Verification items for this drawing (mm, ordinates from the low corner). Give positions to 0.01 mm unless a question says otherwise; leave off trailing zeros. Loops run counter-clockwise (first coordinate to the right, second up) from the corner with the lowest first, then second, coordinate; pieces in that order, holes last. Notation, with made-up numbers: M -24,87.5 L -16,87.5 A17 cw -16,95.5 Z; hole C 89.5,17 d5. An arc over 180 degrees is marked long. Answer in a Markdown table with one row per item.
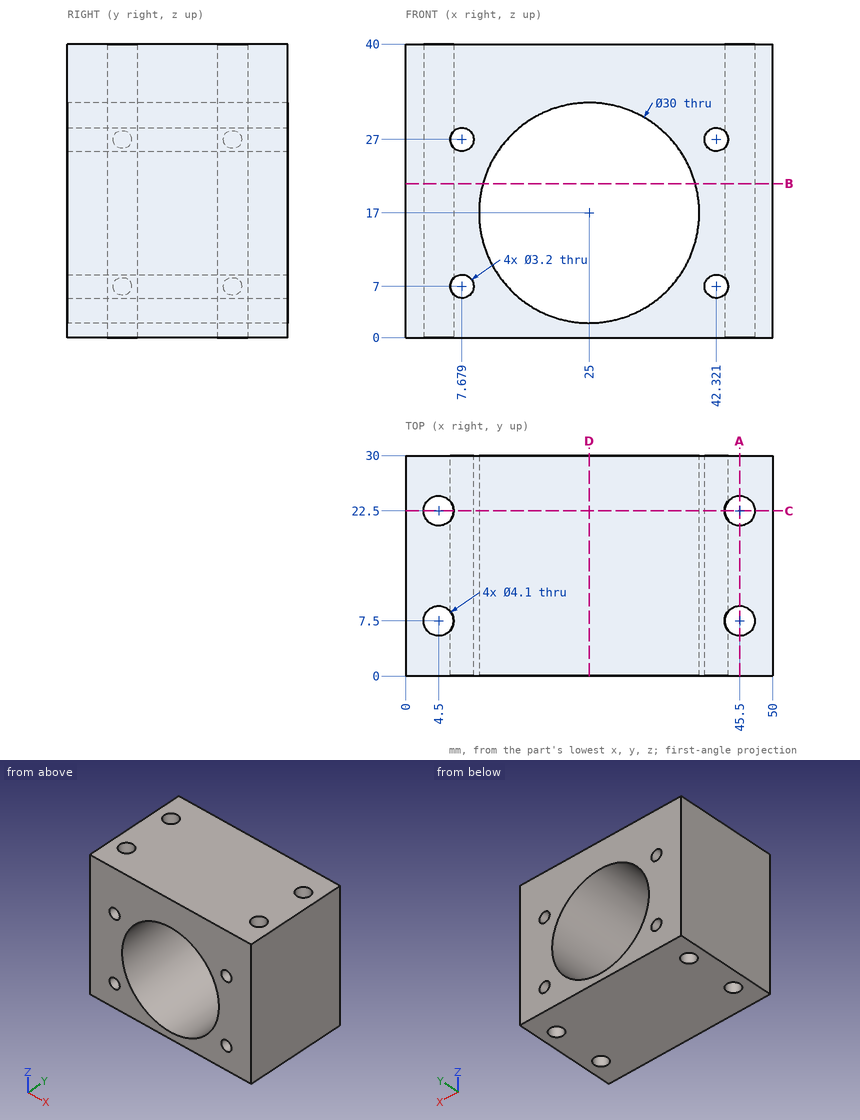
Item 1: Scan lines: L1, parallel to Z at x = 25, y = 4; L2, parallel to X at y = 23.5, z = 17.5; L3, parallel to Y at x = 45, z = 35. Record each from-to range of solid material in increasing order. Write a range as [from, to].
Reported:
| item | result |
|---|---|
| L1 | z = [0, 2], [32, 40] |
| L2 | x = [0, 2.71], [6.29, 10.01], [39.99, 43.71], [47.29, 50] |
| L3 | y = [0, 5.51], [9.49, 20.51], [24.49, 30] |
Item 2: Sectioned sample at A-A (x = 45.5). Record the cut outline in (y, z), and give its area (3 significant figures).
Reported:
| item | result |
|---|---|
| outline | M 0,0 L 5.45,0 L 5.45,40 L 0,40 Z; M 9.55,0 L 20.45,0 L 20.45,40 L 9.55,40 Z; M 24.55,0 L 30,0 L 30,40 L 24.55,40 Z |
| area | 872 mm^2 |
Item 3: Go/stop test with flat-tipped pins: pin 1 (3.5 mm diameter, centred on x = 42.32, z = 7, fed in from -Y); pin 2 (3 mm diameter, centred on x = 42.32, z = 27, fed in from +Y). Record where each tip stops, or that it passes through.
Reported:
| item | result |
|---|---|
| pin 1 | stops at y = 0 |
| pin 2 | passes through |
Item 4: Sectioned sample at C-C (y = 22.5). Record the cut outline in (x, z).
Reported:
| item | result |
|---|---|
| outline | M 0,0 L 2.45,0 L 2.45,40 L 0,40 Z; M 6.55,0 L 43.45,0 L 43.45,5.87 A1.6 cw long 43.45,8.13 L 43.45,25.87 A1.6 cw long 43.45,28.13 L 43.45,40 L 6.55,40 L 6.55,28.13 A1.6 cw long 6.55,25.87 L 6.55,8.13 A1.6 cw long 6.55,5.87 Z; M 47.55,0 L 50,0 L 50,40 L 47.55,40 Z; hole C 25,17 d30 |
Item 5: Sectioned sample at D-D (x = 25). Record the cut outline in (y, z), and give its area (3 significant figures).
Reported:
| item | result |
|---|---|
| outline | M 0,0 L 30,0 L 30,2 L 0,2 Z; M 0,32 L 30,32 L 30,40 L 0,40 Z |
| area | 300 mm^2 |
Item 6: Sectioned sample at B-B (z = 21). Record the cut outline in (x, y).
Reported:
| item | result |
|---|---|
| outline | M 0,0 L 10.54,0 L 10.54,30 L 0,30 Z; M 39.46,0 L 50,0 L 50,30 L 39.46,30 Z; hole C 4.5,7.5 d4.1; hole C 4.5,22.5 d4.1; hole C 45.5,7.5 d4.1; hole C 45.5,22.5 d4.1 |
